Input: dimensioned drawing with shaded views. Units: mm. Origin: part minimum x, y, z. Give positions to 0.01 mm unless a question says otherwise; leave off trailing zeros. Write each loop counter-clockwise with the first axis right and the second up, starting at its lowest first coordinate (ties: lowest second). Pieces come first, ordered by that corner, then holes. Notation, with made-up numbers: (-2.75, 15.25) - (32.25, 15.25) arc R21 cw to (32.25, 48.25) - close; hole circle Ø5 at (-39, 49.25). An arc over 180 degrees is marked (long way). Answer as a JSON object with one key per item and string values. Group by question number.
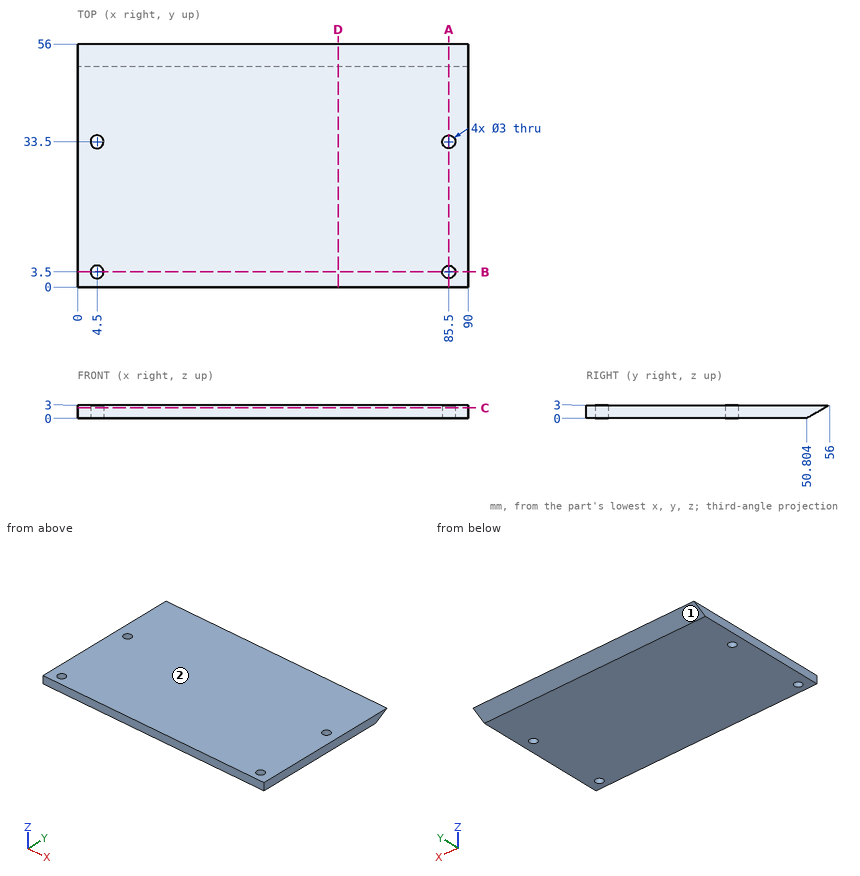
Q1. Section B-B on y = 3.5. Return the cut outline in (x, z).
Q2. Section D-D on x = 60. Return the cut outline in (y, z), then the cut area to 3 significant figures.
Q3. Section C-C on z = 2.4. Return the cut outline in (x, y).
Q4. Draft query along Z for the marked faces 1 and 2. Return one class per face: released by +Z, released by -Z, zero draft, split by the parting line, or undercut.
Q5. Section A-A on x = 85.5. Return the cut outline in (y, z).
Q6. Ray query, probe 1 along X at (y, z) = (33.5, 1.8); probe 2 along X at (y, z) = (33, 0.7); probe 3 along Y at (x, z) = (85.5, 0.7) (1 decimal). Return the intervals inside material, ascending. Write a range as [from, to].
Taken from the geometry:
{
 "1": {"outline": "(0, 0) - (3, 0) - (3, 3) - (0, 3) - close; (6, 0) - (84, 0) - (84, 3) - (6, 3) - close; (87, 0) - (90, 0) - (90, 3) - (87, 3) - close"},
 "2": {"outline": "(0, 0) - (50.8, 0) - (56, 3) - (0, 3) - close", "area": "160 mm²"},
 "3": {"outline": "(0, 0) - (90, 0) - (90, 54.96) - (0, 54.96) - close; hole circle Ø3 at (4.5, 3.5); hole circle Ø3 at (4.5, 33.5); hole circle Ø3 at (85.5, 3.5); hole circle Ø3 at (85.5, 33.5)"},
 "4": {"face 1": "released by -Z", "face 2": "released by +Z"},
 "5": {"outline": "(0, 0) - (2, 0) - (2, 3) - (0, 3) - close; (5, 0) - (32, 0) - (32, 3) - (5, 3) - close; (35, 0) - (50.8, 0) - (56, 3) - (35, 3) - close"},
 "6": {"probe 1": "x = [0, 3], [6, 84], [87, 90]", "probe 2": "x = [0, 3.09], [5.91, 84.09], [86.91, 90]", "probe 3": "y = [0, 2], [5, 32], [35, 52]"}
}
